Build history of the part. All positions in model axes, mm. A direction names the side the tool comes from. Give positions to 0.01 mm unless a question says otherwise; leave off trailing zeros. Order: outer loops, then holes, each group sorted by start corner. A loop starts at its lowest first (then second) coordinate and runs counter-clockwise, first axis right, second up. Notation, with made-up numbers: M 29.5,-11.75 L 54.5,-11.75 A20 ccw 54.5,-7.75 Z; hole C -35.75,3 d5. An arc over 180 degrees is marked long. Answer as CSV lines item,"result".
from build123d import *

# Parameters (mm, degrees)
F0_W     = 1320.8
F0_H     = 558.8
F1_DEPTH = 38.1
F2_W     = 38.1
F2_H     = 342.9
F3_DEPTH = 342.9
F5_DEPTH = 148.844
F6_W     = 508
F6_H     = 203.2
F7_DEPTH = 25.4


with BuildPart() as f1:
    # F0 (on Top) → F1 (new body)
    with BuildSketch(Plane.XY):
        with Locations((0.016812, -382.564251)):
            Rectangle(F0_W, F0_H)
    extrude(amount=F1_DEPTH)

    # F2 (on face) → F3 (join)
    with BuildSketch(Plane.XY.offset(38.1)):
        Polygon((-609.583188, -103.164251), (-660.383188, -103.164251), (-660.383188, -661.964251), (-609.583188, -661.964251), (-609.583188, -319.064251), (-609.583188, -300.014251), align=None)
        Polygon((609.616812, -300.014251), (-609.583188, -300.014251), (-609.583188, -319.064251), (-241.283188, -319.064251), (-203.183188, -319.064251), (203.216812, -319.064251), (241.316812, -319.064251), (609.616812, -319.064251), align=None)
        Polygon((609.616812, -103.164251), (609.616812, -300.014251), (609.616812, -319.064251), (609.616812, -661.964251), (660.416812, -661.964251), (660.416812, -103.164251), align=None)
        with Locations((-222.233188, -490.514251)):
            Rectangle(F2_W, F2_H)
        with Locations((222.266812, -490.514251)):
            Rectangle(F2_W, F2_H)
    extrude(amount=F3_DEPTH)

    # F4 (on face) → F5 (cut)
    with BuildSketch(Plane.YZ.offset(660.416812)):
        with BuildLine():
            Line((-223.814251, 114.3), (-287.314251, 114.3))
            ThreePointArc((-287.314251, 114.3), (-291.804379, 112.440128), (-293.664251, 107.95))
            Line((-293.664251, 107.95), (-293.664251, 44.45))
            ThreePointArc((-293.664251, 44.45), (-291.804379, 39.959872), (-287.314251, 38.1))
            Line((-287.314251, 38.1), (-223.814251, 38.1))
            ThreePointArc((-223.814251, 38.1), (-219.324123, 39.959872), (-217.464251, 44.45))
            Line((-217.464251, 44.45), (-217.464251, 107.95))
            ThreePointArc((-217.464251, 107.95), (-219.324123, 112.440128), (-223.814251, 114.3))
        make_face()
    extrude(amount=-F5_DEPTH, mode=Mode.SUBTRACT)

    # F6 (on face) → F7 (cut)
    with BuildSketch(Plane(origin=(0, -300.014251, 0), x_dir=(-1, 0, 0), z_dir=(0, 1, 0))):
        with Locations((-320.029565, 139.7)):
            Rectangle(F6_W, F6_H)
    extrude(amount=-F7_DEPTH, mode=Mode.SUBTRACT)


solid = f1.part
Item 1: Band-saw the part on C-C (y = -255). Give the cut face in (x, z), and give its area (3 significant figures).
Geometry says:
outline,"M -660.38,0 L 660.42,0 L 660.42,38.1 L -609.58,38.1 L -609.58,381 L -660.38,381 Z; M 609.62,114.3 L 660.42,114.3 L 660.42,381 L 609.62,381 Z"
area,"81,300 mm2"
Item 2: Probe line 1 along X through (y, z) = (-329.5, 259); line 2 along X through (y, z) = (-140.5, 240); line 3 along Y through (x, z) = (-373, 353.5). List the from-to ranges inside material, lowest first. Write a range as from..to.
Geometry says:
line 1,"x = -660.38..-609.58, -241.28..-203.18, 203.22..241.32, 609.62..660.42"
line 2,"x = -660.38..-609.58, 609.62..660.42"
line 3,"y = -319.06..-300.01"
Item 3: Band-saw the part on B-B (x = 166). Give the cut face in (y, z).
Geometry says:
outline,"M -661.96,0 L -103.16,0 L -103.16,38.1 L -661.96,38.1 Z; M -319.06,241.3 L -300.01,241.3 L -300.01,381 L -319.06,381 Z"
Item 4: Band-saw the part on D-D (x = -38). Give the cut face in (y, z).
Geometry says:
outline,"M -661.96,0 L -103.16,0 L -103.16,38.1 L -300.01,38.1 L -300.01,381 L -319.06,381 L -319.06,38.1 L -661.96,38.1 Z"
Item 5: Pull direction Y, two halves, no side cores. Call faces 4 (the flat face through (635, -293.664, 77)), 5 (the flat face through (-9, -379, 0)), 6 (the flat face through (223, -325.414, 141)), 7 (the flat face through (635, -255, 114.3)): released by +Y, released by -Y, zero draft, split by the parting line, or undercut.
Geometry says:
face 4,"undercut"
face 5,"zero draft"
face 6,"released by +Y"
face 7,"undercut"
Item 6: Drop a flat-ended pin along its axis: pin 1 (4 mm diameter, centred on x = -128.5, z = 115.5, fed in from +Y). Give the stop position or say it passes through.
Geometry says:
pin 1,"stops at y = -300.01"
Item 7: Band-saw the part on A-A (z = 208). Give the cut face in (x, y).
Geometry says:
outline,"M -660.38,-661.96 L -609.58,-661.96 L -609.58,-319.06 L -241.28,-319.06 L -241.28,-661.96 L -203.18,-661.96 L -203.18,-319.06 L 66.03,-319.06 L 66.03,-300.01 L -609.58,-300.01 L -609.58,-103.16 L -660.38,-103.16 Z; M 203.22,-661.96 L 241.32,-661.96 L 241.32,-325.41 L 203.22,-325.41 Z; M 574.03,-319.06 L 609.62,-319.06 L 609.62,-661.96 L 660.42,-661.96 L 660.42,-103.16 L 609.62,-103.16 L 609.62,-300.01 L 574.03,-300.01 Z"
Item 8: 3-axis set-ups, long thin cutter, end or side, ignore diameter. For faces 1 (the flat face through (-48, -319.064, 207)), 2 (the flat face through (-609.583, -203, 207)), 3 (the flat face through (635, -217.464, 76)): which of +Z, -Z, +X, -X, +Y, -Y reach the whole face in a straight line?
Geometry says:
face 1,"+Z, -Y"
face 2,"+Z, +Y"
face 3,"+X"
